Verification items for the finished model (mm, model axes). Round coordinates to 2 decimals unless told otherwise and drop trailing zeros. Write each loop counter-clockwise with the first axis right and the second up, starting at its lowest first coordinate (ties: lowest second). Pieces come first, ordered by that corner, then holes.
from build123d import *

# Parameters (mm, degrees)
SKETCH1_W           = 10
SKETCH1_H           = 28.6
BOSS_EXTRUDE1_DEPTH = 4
SKETCH2_R           = 0.935
BOSS_EXTRUDE2_DEPTH = 3


with BuildPart() as part:
    # Sketch1 → Boss-Extrude1 (new body)
    with BuildSketch(Plane(origin=(0, 0, 0), x_dir=(1, 0, 0), z_dir=(0, 1, 0))):
        Rectangle(SKETCH1_W, SKETCH1_H)
    extrude(amount=BOSS_EXTRUDE1_DEPTH)

    # Sketch2 → Boss-Extrude2 (add)
    with BuildSketch(Plane.XZ):
        with Locations(Location((0, 12.8, 0), (0, 0, 270))):
            Circle(SKETCH2_R)
        with Locations(Location((0, -12.8, 0), (0, 0, 90))):
            Circle(SKETCH2_R)
    extrude(amount=BOSS_EXTRUDE2_DEPTH)


solid = part.part
Q1. Sectioned sample at A-A (z = -12.8). Enter the section's corners in (x, y) (3 decimals).
Recorded:
outline: (-5, 0) - (-0.935, 0) - (-0.935, -3) - (0.935, -3) - (0.935, 0) - (5, 0) - (5, 4) - (-5, 4) - close
Q2. Sectioned sample at C-C (x = 0). Enter the section's corners in (y, z) (3 decimals).
Recorded:
outline: (-3, -13.735) - (0, -13.735) - (0, -14.3) - (4, -14.3) - (4, 14.3) - (0, 14.3) - (0, 13.735) - (-3, 13.735) - (-3, 11.865) - (0, 11.865) - (0, -11.865) - (-3, -11.865) - close
Q3. Release check for a two-part mould opening along Z. For faces 1 (the flat face through (0, 2, -14.3)), 2 (the cylindrical face through (0.28, -1.48, 11.91)), 3 (the cylindrical face through (-0.28, -1.48, -11.91)), 4 (the flat face through (0, 2, 14.3)) record: released by +Z, released by -Z, zero draft, split by the parting line, or undercut.
Recorded:
face 1: released by -Z
face 2: undercut
face 3: undercut
face 4: released by +Z
Q4. Material ranges on line 1 along Y through (x, z) = (3.25, 1.5), recorded low to high.
Recorded:
line 1: y = 0 to 4
Q5. Sectioned sample at B-B (y = -0.25). Enter the section's corners in (x, z) (3 decimals).
Recorded:
outline: circle Ø1.87 at (0, -12.8); circle Ø1.87 at (0, 12.8)
Q6. Sectioned sample at D-D (z = 7.75). Enter the section's corners in (x, y).
Recorded:
outline: (-5, 0) - (5, 0) - (5, 4) - (-5, 4) - close
